```python
from build123d import *

# Parameters (mm, degrees)
SKETCH1_R           = 7.5
BOSS_EXTRUDE1_DEPTH = 20
CUT_EXTRUDE1_REACH  = 208.155
SKETCH2_R           = 2
FILLET1_R           = 10
SKETCH3_W           = 40
SKETCH3_H           = 4
BOSS_EXTRUDE2_DEPTH = 24
CUT_EXTRUDE2_REACH  = 212.24
SKETCH4_R           = 2
FILLET3_R           = 10
FILLET4_START       = -5.202040929
FILLET4_DEPTH       = 6.202040929
FILLET4_START_2     = -14.898418687
FILLET4_2_DEPTH     = 9.696377758
FILLET4_START_3     = 20
FILLET4_3_DEPTH     = 5


with BuildPart() as part:
    # Sketch1 → Boss-Extrude1 (new body)
    with BuildSketch(Plane(origin=(0, 0, 0), x_dir=(1, 0, 0), z_dir=(0, 1, 0))):
        with BuildLine():
            Line((10.356157589, -5), (125, -5))
            Line((125, -5), (125, -40))
            Line((125, -40), (105, -40))
            Line((105, -40), (105, -48))
            ThreePointArc((105, -48), (130, -50), (155, -48))
            Line((155, -48), (155, -40))
            Line((155, -40), (135, -40))
            Line((135, -40), (135, 5))
            Line((135, 5), (10.356157589, 5))
            ThreePointArc((10.356157589, 5), (8.131727984, 8.131727984), (5, 10.356157589))
            Line((5, 10.356157589), (5, 140))
            Line((5, 140), (1, 140))
            Line((1, 140), (1, 110))
            Line((1, 110), (-5, 110))
            Line((-5, 110), (-5, 10.356157589))
            ThreePointArc((-5, 10.356157589), (-8.131727984, -8.131727984), (10.356157589, -5))
        make_face()
        with Locations(Location((0, 0, 0), (0, 0, 270))):
            Circle(SKETCH1_R, mode=Mode.SUBTRACT)
    extrude(amount=BOSS_EXTRUDE1_DEPTH)

    # Sketch2 → Cut-Extrude1 (cut, up to next)
    with BuildSketch(Plane(origin=(5, 0, 0), x_dir=(0, 0, -1), z_dir=(1, 0, 0)), mode=Mode.PRIVATE) as cut_extrude1_sk1:
        with Locations((135.656854249, 4.343145751)):
            Circle(SKETCH2_R)
    cut_extrude1_tool1 = extrude(cut_extrude1_sk1.sketch, amount=-CUT_EXTRUDE1_REACH, mode=Mode.PRIVATE) & part.part
    # Sketch2 → Cut-Extrude1 (cut, up to next)
    with BuildSketch(Plane(origin=(5, 0, 0), x_dir=(0, 0, -1), z_dir=(1, 0, 0)), mode=Mode.PRIVATE) as cut_extrude1_sk2:
        with Locations((124.343145751, 4.343145751)):
            Circle(SKETCH2_R)
    cut_extrude1_tool2 = extrude(cut_extrude1_sk2.sketch, amount=-CUT_EXTRUDE1_REACH, mode=Mode.PRIVATE) & part.part
    # Sketch2 → Cut-Extrude1 (cut, up to next)
    with BuildSketch(Plane(origin=(5, 0, 0), x_dir=(0, 0, -1), z_dir=(1, 0, 0)), mode=Mode.PRIVATE) as cut_extrude1_sk3:
        with Locations((124.343145751, 15.656854249)):
            Circle(SKETCH2_R)
    cut_extrude1_tool3 = extrude(cut_extrude1_sk3.sketch, amount=-CUT_EXTRUDE1_REACH, mode=Mode.PRIVATE) & part.part
    # Sketch2 → Cut-Extrude1 (cut, up to next)
    with BuildSketch(Plane(origin=(5, 0, 0), x_dir=(0, 0, -1), z_dir=(1, 0, 0)), mode=Mode.PRIVATE) as cut_extrude1_sk4:
        with Locations((135.656854249, 15.656854249)):
            Circle(SKETCH2_R)
    cut_extrude1_tool4 = extrude(cut_extrude1_sk4.sketch, amount=-CUT_EXTRUDE1_REACH, mode=Mode.PRIVATE) & part.part
    add(cut_extrude1_tool1.solids().sort_by_distance((5, 4.343146, -135.656854))[0], mode=Mode.SUBTRACT)
    add(cut_extrude1_tool2.solids().sort_by_distance((5, 4.343146, -124.343146))[0], mode=Mode.SUBTRACT)
    add(cut_extrude1_tool3.solids().sort_by_distance((5, 15.656854, -124.343146))[0], mode=Mode.SUBTRACT)
    add(cut_extrude1_tool4.solids().sort_by_distance((5, 15.656854, -135.656854))[0], mode=Mode.SUBTRACT)

    # Fillet1
    # the kernel refuses this fillet: 10 mm, written as the material it adds along each edge
    with BuildSketch(Plane(origin=(1, 0, -110), x_dir=(0, 0, -1), z_dir=(0, 1, 0))) as fillet1_piece_1:
        with BuildLine():
            CenterArc((9.16515139, 10), FILLET1_R, 203.578178478, 66.421821522)
            Line((0, 6), (0, 0))
            Line((0, 0), (9.16515139, 0))
        make_face()
    extrude(amount=20)
    with BuildSketch(Plane(origin=(125, 0, 40), x_dir=(0, 0, -1), z_dir=(0, 1, 0)), Plane(origin=(135, 0, 40), x_dir=(1, 0, 0), z_dir=(0, 1, 0)), Plane(origin=(125, 0, 5), x_dir=(-1, 0, 0), z_dir=(0, 1, 0))) as fillet1_piece_2:
        with BuildLine():
            CenterArc((FILLET1_R, FILLET1_R), FILLET1_R, 180, 90)
            Line((0, FILLET1_R), (0, 0))
            Line((0, 0), (FILLET1_R, 0))
        make_face()
    extrude(amount=20)
    with BuildSketch(Plane(origin=(10.356157589, 0, 5), x_dir=(1, 0, 0), z_dir=(0, 1, 0))) as fillet1_piece_3:
        with BuildLine():
            CenterArc((5.046764212, -10), FILLET1_R, 90, 45.75928121)
            ThreePointArc((-2.117385463, -3.023255814), (-0.936610269, -1.597130308), (0, 0))
            Line((0, 0), (5.046764212, 0))
        make_face()
    extrude(amount=20)
    with BuildSketch(Plane(origin=(10.356157589, 0, -5), x_dir=(1, 0, 0), z_dir=(0, 1, 0))) as fillet1_piece_4:
        with BuildLine():
            CenterArc((5.046764212, 10), FILLET1_R, 224.24071879, 45.75928121)
            ThreePointArc((-2.117385463, 3.023255814), (-0.936610269, 1.597130308), (0, 0))
            Line((0, 0), (5.046764212, 0))
        make_face()
    extrude(amount=20)
    with BuildSketch(Plane(origin=(5, 0, -10.356157589), x_dir=(0.8190910712491061, 0, 0.5736635050271124), z_dir=(0, 1, 0))) as fillet1_piece_5:
        with BuildLine():
            CenterArc((5.295766266, 9.870394555), FILLET1_R, 215.006090265, 45.75928121)
            Line((-2.895144447, 4.133759505), (0, 0))
            ThreePointArc((0, 0), (1.845494305, 0.149046262), (3.690988609, 0))
        make_face()
    extrude(amount=20)
    with BuildSketch(Plane(origin=(-5, 0, -10.356157589), x_dir=(-0.8190910712491065, 0, 0.5736635050271119), z_dir=(0, 1, 0))) as fillet1_piece_6:
        with BuildLine():
            CenterArc((5.295766266, -9.870394555), FILLET1_R, 99.234628525, 45.75928121)
            Line((-2.895144447, -4.133759505), (0, 0))
            ThreePointArc((0, 0), (1.845494305, -0.149046262), (3.690988609, 0))
        make_face()
    extrude(amount=20)
    # the kernel refuses this fillet: 10 mm, written as the material it takes off along each edge
    with BuildSketch(Plane(origin=(135, -25, -5), x_dir=(0, 0, 1), z_dir=(0, 1, 0))) as fillet1_2_piece_1:
        with BuildLine():
            CenterArc((FILLET1_R, -FILLET1_R), FILLET1_R, 90, 90)
            Line((0, -FILLET1_R), (0, 0))
            Line((0, 0), (FILLET1_R, 0))
        make_face()
    extrude(amount=70, mode=Mode.SUBTRACT)

    # Sketch3 → Boss-Extrude2 (add)
    with BuildSketch(Plane(origin=(5, 0, 0), x_dir=(0, 0, -1), z_dir=(1, 0, 0))):
        with Locations((120, 22)):
            Rectangle(SKETCH3_W, SKETCH3_H)
    extrude(amount=-BOSS_EXTRUDE2_DEPTH)

    # Sketch4 → Cut-Extrude2 (cut, up to next)
    with BuildSketch(Plane(origin=(0, 24, 0), x_dir=(1, 0, 0), z_dir=(0, 1, 0)), mode=Mode.PRIVATE) as cut_extrude2_sk1:
        with Locations(Location((-3.343145751, 135.656854249, 0), (0, 0, 270))):
            Circle(SKETCH4_R)
    cut_extrude2_tool1 = extrude(cut_extrude2_sk1.sketch, amount=-CUT_EXTRUDE2_REACH, mode=Mode.PRIVATE) & part.part
    # Sketch4 → Cut-Extrude2 (cut, up to next)
    with BuildSketch(Plane(origin=(0, 24, 0), x_dir=(1, 0, 0), z_dir=(0, 1, 0)), mode=Mode.PRIVATE) as cut_extrude2_sk2:
        with Locations(Location((-14.656854249, 135.656854249, 0), (0, 0, 270))):
            Circle(SKETCH4_R)
    cut_extrude2_tool2 = extrude(cut_extrude2_sk2.sketch, amount=-CUT_EXTRUDE2_REACH, mode=Mode.PRIVATE) & part.part
    # Sketch4 → Cut-Extrude2 (cut, up to next)
    with BuildSketch(Plane(origin=(0, 24, 0), x_dir=(1, 0, 0), z_dir=(0, 1, 0)), mode=Mode.PRIVATE) as cut_extrude2_sk3:
        with Locations(Location((-14.656854249, 124.343145751, 0), (0, 0, 270))):
            Circle(SKETCH4_R)
    cut_extrude2_tool3 = extrude(cut_extrude2_sk3.sketch, amount=-CUT_EXTRUDE2_REACH, mode=Mode.PRIVATE) & part.part
    # Sketch4 → Cut-Extrude2 (cut, up to next)
    with BuildSketch(Plane(origin=(0, 24, 0), x_dir=(1, 0, 0), z_dir=(0, 1, 0)), mode=Mode.PRIVATE) as cut_extrude2_sk4:
        with Locations(Location((-3.343145751, 124.343145751, 0), (0, 0, 270))):
            Circle(SKETCH4_R)
    cut_extrude2_tool4 = extrude(cut_extrude2_sk4.sketch, amount=-CUT_EXTRUDE2_REACH, mode=Mode.PRIVATE) & part.part
    add(cut_extrude2_tool1.solids().sort_by_distance((-3.343146, 24, -135.656854))[0], mode=Mode.SUBTRACT)
    add(cut_extrude2_tool2.solids().sort_by_distance((-14.656854, 24, -135.656854))[0], mode=Mode.SUBTRACT)
    add(cut_extrude2_tool3.solids().sort_by_distance((-14.656854, 24, -124.343146))[0], mode=Mode.SUBTRACT)
    add(cut_extrude2_tool4.solids().sort_by_distance((-3.343146, 24, -124.343146))[0], mode=Mode.SUBTRACT)

    # Fillet3
    # the kernel refuses this fillet: 10 mm, written as the material it adds along each edge
    with BuildSketch(Plane(origin=(5, 20, -100), x_dir=(0, 0, 1), z_dir=(-1, 0, 0))) as fillet3_piece_1:
        with BuildLine():
            CenterArc((8, 10), FILLET3_R, 216.869897646, 53.130102354)
            Line((0, 4), (0, 0))
            Line((0, 0), (8, 0))
        make_face()
    extrude(amount=10)

    # Fillet4: read off the stored shape, not the designer's step
    # Fillet4 outline → Fillet4 (add)
    with BuildSketch(Plane.YZ.offset(FILLET4_START)):
        with BuildLine():
            Line((20, -92), (20, -100))
            Line((20, -100), (24.000002869, -100.000002152))
            ThreePointArc((24.000002869, -100.000002152), (21.055728892, -96.472137559), (20, -92))
        make_face()
    extrude(amount=FILLET4_DEPTH)

    # Fillet4 2 outline → Fillet4 2 (add)
    with BuildSketch(Plane.YZ.offset(FILLET4_START_2)):
        with BuildLine():
            ThreePointArc((24.000002869, -100.000002152), (21.055728892, -96.472137559), (20, -92))
            Line((20, -92), (20, -100))
            Line((20, -100), (24.000002869, -100.000002152))
        make_face()
    extrude(amount=FILLET4_2_DEPTH)

    # Fillet4 3 outline → Fillet4 3 (cut)
    with BuildSketch(Plane(origin=(0, 0, 0), x_dir=(1, 0, 0), z_dir=(0, 1, 0)).offset(FILLET4_START_3)):
        with BuildLine():
            Line((-4.793792738, 90), (-5.202041029, 92))
            ThreePointArc((-5.202041029, 92), (-8.636183479, 97.713743532), (-14.898418687, 99.999484049))
            Line((-14.898418687, 99.999484049), (-14.898418687, 90))
            Line((-14.898418687, 90), (-4.793792738, 90))
        make_face()
    extrude(amount=FILLET4_3_DEPTH, mode=Mode.SUBTRACT)


solid = part.part
```
The model under review builds one solid part; all positions refer to its coordinate system, in mm. A direction names the side the tool comes from. Round coordinates to 2 decimals unless told otherwise and drop trailing zeros. Order: outer loops, then holes, each group sorted by start corner. A loop starts at its lowest first (then second) coordinate and runs counter-clockwise, first axis right, second up. Notation, with made-up numbers: M -9,72.5 L 39,72.5 A21 cw 39,79.5 Z; hole C 1.25,84 d1. An arc over 180 degrees is marked long. Use a Markdown table: item, result.
1) Consider section B-B (y = 8.5). Write out the cut boundary in (x, z).
Report:
| item | result |
|---|---|
| outline | M -8.02,-8.24 A10 cw -5,-15.4 L -5,-110 A10 cw 1,-119.17 L 1,-140 L 5,-140 L 5,-15.4 A10 cw 8.02,-8.24 A11.5 ccw 8.24,-8.02 A10 cw 15.4,-5 L 125,-5 A10 ccw 135,5 L 135,30 A10 cw 145,40 L 155,40 L 155,48 A157.25 ccw 105,48 L 105,40 L 115,40 A10 cw 125,30 L 125,15 A10 cw 115,5 L 15.4,5 A10 cw 8.24,8.02 A11.5 ccw long Z; hole C 0,0 d15 |
2) Consider section A-A (z = 0). Write out the cut boundary in (x, y).
Report:
| item | result |
|---|---|
| outline | M -11.5,0 L -7.5,0 L -7.5,20 L -11.5,20 Z; M 7.5,0 L 133.66,0 L 133.66,20 L 7.5,20 Z |
3) Wall thickness on line 1 along Z through (x, y) = (47.5, 13.5); line 2 along X through (y, z) = (17.25, 27): over which ranges is each line inside the solid? List them lowest first. Write a range as [from, to].
Report:
| item | result |
|---|---|
| line 1 | [-5, 5] |
| line 2 | [125, 135] |
4) Consider section D-D (z = -107.5). Write out the cut boundary in (x, y), then the cut area to 3 significant figures.
Report:
| item | result |
|---|---|
| outline | M -19,20 L -5,20 L -5,0 L 5,0 L 5,24 L -19,24 Z |
| area | 296 mm^2 |
5) Tool access review of faces 1 (the face through (5, 10, -77)), 2 (the face through (122.15, 9.86, 8.01)), 3 (the face through (121.99, 9.86, 37.15)): name each direction out of +Z, -Z, +X, -X, +Y, -Y from which nothing blocks a thin tool from reaching the whole face with its end or side.
Report:
| item | result |
|---|---|
| face 1 | -Z, +X, +Y, -Y |
| face 2 | +Y, -Y |
| face 3 | -X, +Y, -Y |
6) Insertion check: pin 1 (24 mm diameter, centred on x = 0, z = 0, fed in from +Y); pin 2 (10 mm diameter, centred on x = 67.5, y = 12.5, fed in from +Z); pin 3 (2.5 mm diameter, centred on y = 10.5, z = 44.5, fed in from -X). Each pin has a flat end and moves straight along its axis. Give the tip position at first contact, or say it passes through.
Report:
| item | result |
|---|---|
| pin 1 | y = 20 |
| pin 2 | z = 5 |
| pin 3 | x = 105 |
7) Draft analysis for pull direction Y (two halves, no side actions). For faces 4 (the face through (3.03, 4.43, -133.66)), 5 (the face through (63, 20, -3)), 6 (the face through (155, 10, 44)), 7 (the face through (3.03, 15.74, -133.66)), state which applies: released by +Y, released by -Y, zero draft, split by the parting line, or undercut.
Report:
| item | result |
|---|---|
| face 4 | undercut |
| face 5 | released by +Y |
| face 6 | zero draft |
| face 7 | undercut |
8) Consider section C-C (x = 100.5). Write out the cut boundary in (y, z), then the cut area to 3 significant figures.
Report:
| item | result |
|---|---|
| outline | M 0,-5 L 20,-5 L 20,5 L 0,5 Z |
| area | 200 mm^2 |
